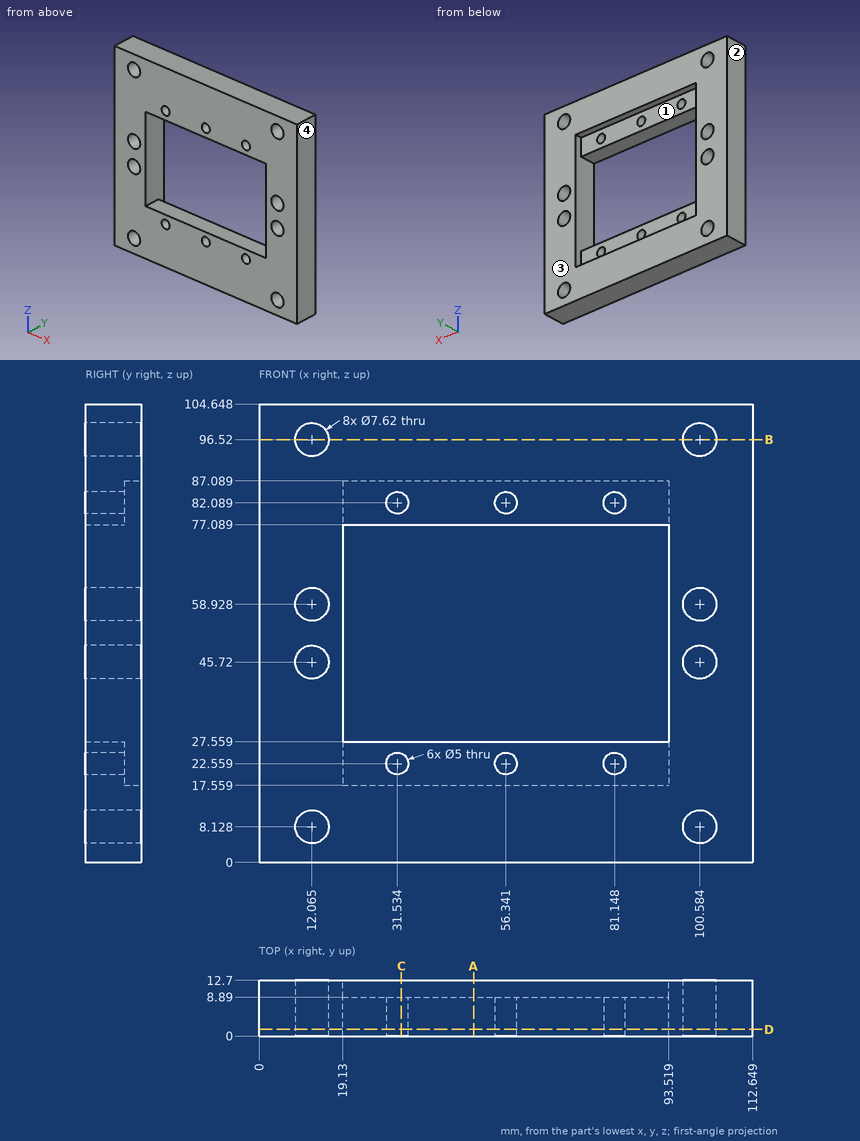
Answer from the drawing. Dimensions are ordinates in mm from the lowest x, y and z of the part. Give positions to 0.01 mm unless a question says otherwise; leave off trailing zeros. Order: outer loops, then holes, each group sorted by start corner. A loop starts at its lowest first (then second) coordinate and runs counter-clockwise, first axis right, second up. Notation, with made-up numbers: (7, 49.25) - (22, 49.25) arc R13 ccw to (22, 64.25) - close; hole circle Ø4 at (-22.75, 75). An arc over 180 degrees is marked (long way). One line per item, written item: value. Start each with the question number.
1. Section B-B, the plane z = 96.52 is taken. Write down the section's boundary in (x, y) (1 decimal).
2. Section C-C, the plane x = 32.5 is taken. Write down the section's boundary in (y, z) (1 decimal), then the cut area to 3 significant figures.
3. Section D-D, the plane y = 1.5 is taken. Count the separate pieces of the cut face and the enclosed holes in it, then the cut area to 3 significant figures.
4. Consider line 1 (Z direction, x = 100.5, y = 11.5); line 2 (X direction, y = 7.5, z = 45.72) (1 decimal); line 3 (X direction, y = 5.5, z = 50.5). Determine where each line is inside the solid, lowest interval first.
5. Section A-A, the plane x = 49 is taken. Write down the section's boundary in (y, z).
6. Each of these flat-tipped pins is pushed along its axis until it touches: pin 1 Ø6.5 at (x, z) = (31.53, 22.56) entering from -Y; pin 2 Ø5 at (x, z) = (58.5, 84.5) entering from +Y. Where does it stop, or does it pass through?
7. For a pull along X with two mould halves and no side action, classify the marked faces 1, 2, 3 and 4 as released by +X, released by -X, zero draft, split by the parting line, or undercut.
Filled sheet:
1. outline: (0, 0) - (8.3, 0) - (8.3, 12.7) - (0, 12.7) - close; (15.9, 0) - (96.8, 0) - (96.8, 12.7) - (15.9, 12.7) - close; (104.4, 0) - (112.6, 0) - (112.6, 12.7) - (104.4, 12.7) - close
2. outline: (0, 0) - (12.7, 0) - (12.7, 17.6) - (8.9, 17.6) - (8.9, 20.3) - (0, 20.3) - close; (0, 24.9) - (8.9, 24.9) - (8.9, 27.6) - (0, 27.6) - close; (0, 77.1) - (8.9, 77.1) - (8.9, 79.8) - (0, 79.8) - close; (0, 84.4) - (8.9, 84.4) - (8.9, 87.1) - (12.7, 87.1) - (12.7, 104.6) - (0, 104.6) - close
2. area: 542 mm²
3. separate pieces: 1
3. enclosed holes: 15
3. area: 7,620 mm²
4. line 1: 0 to 4.32, 11.94 to 41.91, 49.53 to 55.12, 62.74 to 92.71, 100.33 to 104.65
4. line 2: 0 to 8.3, 15.9 to 19.1, 93.5 to 96.8, 104.4 to 112.6
4. line 3: 0 to 19.13, 93.52 to 112.65
5. outline: (0, 0) - (12.7, 0) - (12.7, 17.56) - (8.89, 17.56) - (8.89, 27.56) - (0, 27.56) - close; (0, 77.09) - (8.89, 77.09) - (8.89, 87.09) - (12.7, 87.09) - (12.7, 104.65) - (0, 104.65) - close
6. pin 1: y = 0
6. pin 2: y = 8.89
7. face 1: undercut
7. face 2: released by -X
7. face 3: zero draft
7. face 4: released by +X
